```python
from build123d import *

# Parameters (mm, degrees)
F0_R     = 17.5
F1_DEPTH = 50
F2_W     = 20
F2_H     = 20
F3_DEPTH = 25
F5_DEPTH = 25


with BuildPart() as f1:
    # F0 (on Top) → F1 (new body, symmetric)
    with BuildSketch(Plane.XY):
        Circle(F0_R)
    extrude(amount=F1_DEPTH, both=True)

    # F2 (on face) → F3 (join)
    with BuildSketch(Plane.XY.offset(50)):
        Rectangle(F2_W, F2_H)
    extrude(amount=F3_DEPTH)

    # F4 (on Right) → F5 (cut, symmetric)
    with BuildSketch(Plane.YZ):
        Polygon((41.704226, -61.003525), (28.838029, 24.845071), (-43.478873, -23.514086), (-43.478873, -61.003525), align=None)
    extrude(amount=F5_DEPTH, both=True, mode=Mode.SUBTRACT)


solid = f1.part
```
Geometry check sheet. Reference: the model listing, model coordinates, mm. A direction names the side the tool comes from. Give positions to 0.01 mm unless a question says otherwise; leave off trailing zeros. Loops run counter-clockwise (first coordinate to the right, second up) from the corner with the lowest first, then second, coordinate; pieces in that order, holes last. Notation, with made-up numbers: M -8,-15 L 8,-15 A16 cw 8,13 Z; hole C 44,80.25 d7. An arc over 180 degrees is marked long. Write item = value, one per line. Start each with the question number.
1. Section check D-D, the plane z = 3.5. Enter the section's corners in (x, y).
2. Section check B-B, the plane y = 8.5. Enter the section's corners in (x, z), plus the area to 3 significant figures.
3. Thickness scan on probe 1 along Y at (x, z) = (0, 29.5); probe 2 along X at (y, z) = (-6, 54); probe 3 along X at (y, z) = (0.5, 17). Record the ranges inside material, lowest first.
4. Go/stop test with flat-tipped pins: P1, Ø10, axis at x = -11, z = 24, coming from the +Y side; P2, Ø8, axis at x = 8, z = 21, coming from the +Y side; P3, Ø6, axis at x = 5, z = 68, coming from the -Y side. Record where each tip stops, or that it passes through.
5. Section check A-A, the plane x = 0. Enter the section's corners in (y, z).
6. Tool access check on faces 1 (the face through (0, 10, 62)), 2 (the face through (10, 0, 62)), 3 (the face through (0, -10, 62)), 4 (the face through (-10, 0, 62)). Record the directions out of +Z, -Z, +X, -X, +Y, -Y that give a thin tool (end or side, any length) a straight path to the whole face; none if there is none.
7. Section check C-C, the plane z = 47.5. Enter the section's corners in (x, y), plus the area to 3 significant figures.
Values follow:
q1.outline = M -17.23,-3.08 A17.5 ccw 17.23,-3.08 Z
q2.outline = M -15.3,11.24 L 15.3,11.24 L 15.3,50 L 10,50 L 10,75 L -10,75 L -10,50 L -15.3,50 Z
q2.area = 1,690 mm^2
q3.probe_1 = -17.5 to 17.5
q3.probe_2 = -10 to 10
q3.probe_3 = -17.49 to 17.49
q4.P1 = 16.44
q4.P2 = 17.04
q4.P3 = -10
q5.outline = M -17.5,-6.14 L 17.5,17.26 L 17.5,50 L 10,50 L 10,75 L -10,75 L -10,50 L -17.5,50 Z
q6.face_1 = +Z, +X, -X, +Y
q6.face_2 = +Z, +X, +Y, -Y
q6.face_3 = +Z, +X, -X, -Y
q6.face_4 = +Z, -X, +Y, -Y
q7.outline = C 0,0 d35
q7.area = 962 mm^2
